Geometry: see drawing. Coordinates: mm, zero at the bounding-box minimum. A direction names the side the tool comes from. Give positions to 0.01 mm unless a question says otherwise; leave off trailing zeros. Order: outer loops, then holes, each group sorted by start corner. A loop starts at its lowest first (then second) coordinate and runs counter-clockwise, first axis right, second up. Notation, with made-up numbers: M 1,37 L 19,37 A26 ccw 19,75 Z; hole C 4.25,53.25 d2. An arc over 180 degrees is marked long. Use a Markdown table: item, result.
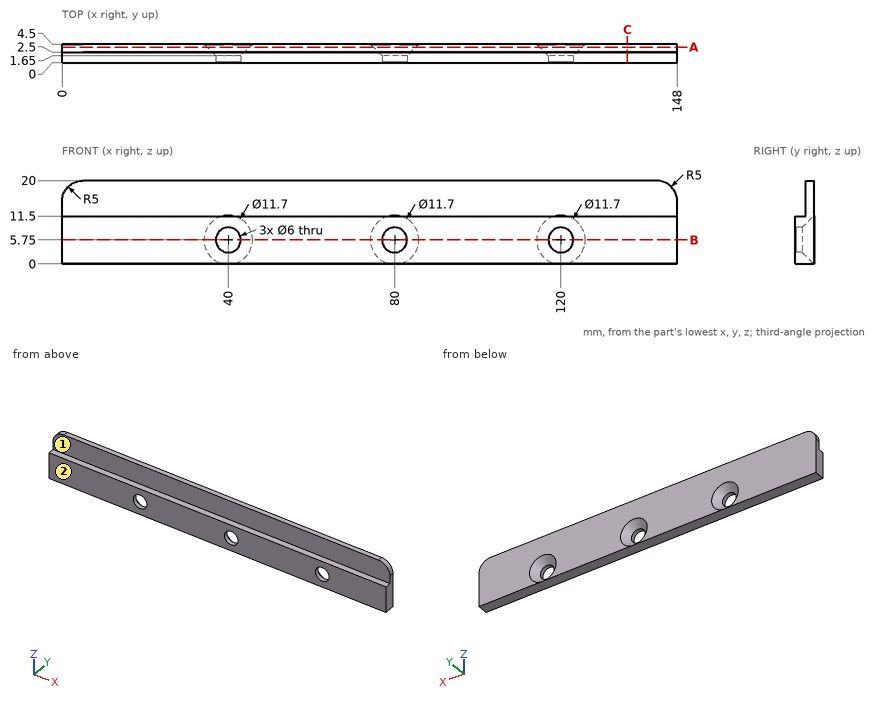
1) First-contact query: pin 1 Ø5 at (x, z) = (80, 5.75) entering from +Y; pin 2 Ø2.5 at (x, z) = (43.5, 17.5) entering from -Y; pin 3 Ø1 at (x, y) = (66, 1) entering from +Z. Flat tips, straight axial feed; report the tip coordinate or a pass-through.
Response values:
| item | result |
|---|---|
| pin 1 | passes through |
| pin 2 | stops at y = 2.5 |
| pin 3 | stops at z = 11.5 |
2) Material intervals for line 1 (Z direction, x = 120, y = 0.7); line 2 (Z direction, x = 114, y = 1.65); line 3 (Y direction, x = 38, z = 12.25), sorted ascending. Write a range as from..to.
Response values:
| item | result |
|---|---|
| line 1 | z = 0..2.75, 8.75..11.5 |
| line 2 | z = 0..11.5 |
| line 3 | y = 2.5..4.5 |
3) Cut plane B-B on z = 5.75. Return loops of the section in (x, y), and give its area (3 significant figures).
Response values:
| item | result |
|---|---|
| outline | M 0,0 L 37,0 L 37,1.65 L 34.15,4.5 L 0,4.5 Z; M 43,0 L 77,0 L 77,1.65 L 74.15,4.5 L 45.85,4.5 L 43,1.65 Z; M 83,0 L 117,0 L 117,1.65 L 114.15,4.5 L 85.85,4.5 L 83,1.65 Z; M 123,0 L 148,0 L 148,4.5 L 125.85,4.5 L 123,1.65 Z |
| area | 561 mm² |
4) Reachability of the marked faces 1 and 2 from +Z, -Z, +X, -X, +Y, -Y: full face, straight path, thin tool, end or side. Return the list, or none.
Response values:
| item | result |
|---|---|
| face 1 | +Z, +X, -X, -Y |
| face 2 | +Z, -Z, +X, -X, -Y |
5) Cut plane C-C on x = 136. Return loops of the section in (y, z).
Response values:
| item | result |
|---|---|
| outline | M 0,0 L 4.5,0 L 4.5,20 L 2.5,20 L 2.5,11.5 L 0,11.5 Z |
6) Cut plane A-A on y = 3.75. Return loops of the section in (x, z), and give its area (3 significant figures).
Response values:
| item | result |
|---|---|
| outline | M 0,0 L 148,0 L 148,15 A5 ccw 143,20 L 5,20 A5 ccw 0,15 Z; hole C 40,5.75 d10.2; hole C 80,5.75 d10.2; hole C 120,5.75 d10.2 |
| area | 2,700 mm² |
